Autodesk Inventor part; units mm, degrees
ref_plane "Piano di lavoro1" through (0, 13.85, 0) normal (0, 1, 0) x (1, 0, 0)
ref_plane "Piano di lavoro2" through (0, -10.75, 0) normal (0, -1, 0) x (1, 0, 0)
ref_plane "YZ Plane" through (0, 0, 0) normal (1, 0, 0) x (0, 1, 0)
sketch "Schizzo1" plane through (0, 0, 0) normal (0, 1, 0) x (-1, 0, 0)
  line L0 (-8.85, -43.18) -> (8.95, -43.18)
  line L1 (8.95, -43.18) -> (8.95, 17.78)
  line L2 (8.95, 17.78) -> (-8.85, 17.78)
  line L3 (-8.85, 17.78) -> (-8.85, -43.18)
  line L4 (-8.85, 17.78) -> (8.95, -43.18) construction
  line L5 (8.95, 17.78) -> (-8.85, -43.18) construction
  line L6 (8.95, 16.48) -> (-8.95, 16.48) construction
  line L7 (-7.6, 17.78) -> (-7.6, -43.18) construction
  circle A0 centre (-7.6, 16.48) radius 0.425
  circle A1 centre (-7.6, 13.94) radius 0.425
  circle A2 centre (-7.6, 11.4) radius 0.425
  circle A3 centre (-7.6, 8.86) radius 0.425
  circle A4 centre (-7.6, 6.32) radius 0.425
  circle A5 centre (-7.6, 3.78) radius 0.425
  circle A6 centre (-7.6, 1.24) radius 0.425
  circle A7 centre (-7.6, -1.3) radius 0.425
  circle A8 centre (-7.6, -3.84) radius 0.425
  circle A9 centre (-7.6, -6.38) radius 0.425
  circle A10 centre (-7.6, -8.92) radius 0.425
  circle A11 centre (-7.6, -11.46) radius 0.425
  circle A12 centre (-7.6, -14) radius 0.425
  circle A13 centre (-7.6, -16.54) radius 0.425
  circle A14 centre (-5.06, 16.48) radius 0.425
  circle A15 centre (-2.52, 16.48) radius 0.425
  circle A16 centre (0.02, 16.48) radius 0.425
  circle A17 centre (2.56, 16.48) radius 0.425
  circle A18 centre (5.1, 16.48) radius 0.425
  circle A19 centre (7.64, 16.48) radius 0.425
  circle A20 centre (7.64, 13.94) radius 0.425
  circle A21 centre (7.64, 11.4) radius 0.425
  circle A22 centre (7.64, 8.86) radius 0.425
  circle A23 centre (7.64, 6.32) radius 0.425
  circle A24 centre (7.64, 3.78) radius 0.425
  circle A25 centre (7.64, 1.24) radius 0.425
  circle A26 centre (7.64, -1.3) radius 0.425
  circle A27 centre (7.64, -3.84) radius 0.425
  circle A28 centre (7.64, -6.38) radius 0.425
  circle A29 centre (7.64, -8.92) radius 0.425
  circle A30 centre (7.64, -11.46) radius 0.425
  circle A31 centre (7.64, -14) radius 0.425
  circle A32 centre (7.64, -16.54) radius 0.425
  circle A33 centre (7.64, -19.08) radius 0.425
  circle A34 centre (7.64, -21.62) radius 0.425
  circle A35 centre (7.64, -24.16) radius 0.425
  circle A36 centre (7.64, -26.7) radius 0.425
  circle A37 centre (7.64, -29.24) radius 0.425
  circle A38 centre (7.64, -31.78) radius 0.425
  circle A39 centre (7.64, -34.32) radius 0.425
  circle A40 centre (7.64, -36.86) radius 0.425
  circle A41 centre (7.64, -39.4) radius 0.425
  circle A42 centre (7.64, -41.94) radius 0.425
  circle A43 centre (-7.6, -19.08) radius 0.425
  circle A44 centre (-7.6, -21.62) radius 0.425
  circle A45 centre (-7.6, -24.16) radius 0.425
  circle A46 centre (-7.6, -26.7) radius 0.425
  circle A47 centre (-7.6, -29.24) radius 0.425
  circle A48 centre (-7.6, -31.78) radius 0.425
  circle A49 centre (-7.6, -34.32) radius 0.425
  circle A50 centre (-7.6, -36.86) radius 0.425
  circle A51 centre (-7.6, -39.4) radius 0.425
  circle A52 centre (-7.6, -41.94) radius 0.425
  circle A53 centre (-5.06, -29.24) radius 0.425
  circle A54 centre (-2.52, -29.24) radius 0.425
  circle A55 centre (0.02, -29.24) radius 0.425
  circle A56 centre (2.56, -29.24) radius 0.425
  circle A57 centre (5.1, -29.24) radius 0.425
  point P0 (0, 0)
  point P1 (0.05, -12.7)
  dimension "d0" = 17.8
  dimension "d1" = 60.96
  dimension "d4" = 1.3
  dimension "d5" = 1.25
  dimension "d6" = 0.85
  dimension "d9" = 2.54
  dimension "d16" = 2.54
  dimension "d23" = 2.54
  dimension "d166" = 2.54
  dimension "d169" = 2.54
extrude "Estrusione2" add sketch "Schizzo1" along normal blind 1.6 contours L3 L2 L1 L0 | A14 | A15 | A16 | A17 | A18
fillet "Raccordo1" radius 0.2 12 edges at (-0.05, 0, 17.78) (-0.05, 1.6, 17.78) (8.85, 0.8, 17.78) (8.85, 0, -12.7) (8.85, 1.6, -12.7) (8.85, 0.8, -43.18) (-0.05, 0, -43.18) (-8.95, 0, -12.7) (-8.95, 0.8, -43.18) (-8.95, 0.8, 17.78) (-8.95, 1.6, -12.7) (-0.05, 1.6, -43.18)
ref_plane "Piano di lavoro1" through (0, 13.85, 0) normal (0, 1, 0) x (1, 0, 0)
sketch "Schizzo2" plane through (0, 13.85, 0) normal (0, 1, 0) x (1, 0, 0)
  line L0 (-8.9159, -19.3191) -> (-8.9159, 43.0633) construction
  line L1 (-8.9159, 43.0633) -> (8.8631, 43.0633) construction
  line L2 (8.8631, 43.0633) -> (8.8631, -19.3191) construction
  line L3 (8.8631, -19.3191) -> (-8.9159, -19.3191) construction
decal "Decalcomania1"
ref_plane "Piano di lavoro2" through (0, -10.75, 0) normal (0, -1, 0) x (1, 0, 0)
sketch "Schizzo3" plane through (0, -10.75, 0) normal (0, -1, 0) x (1, 0, 0)
  line L0 (9.0474, 17.6328) -> (9.0474, -44.6653) construction
  line L1 (9.0474, -44.6653) -> (-9.0191, -44.6653) construction
  line L2 (-9.0191, -44.6653) -> (-9.0191, 17.6328) construction
  line L3 (-9.0191, 17.6328) -> (9.0474, 17.6328) construction
  point P0 (0, 0)
decal "Decalcomania2"
sketch "Schizzo4" plane through (0, 1.6, 0) normal (0, 1, 0) x (1, 0, 0)
  circle A0 centre (7.6, 11.46) radius 0.425
sketch "Schizzo5" plane through (0, 1.6, 0) normal (0, 1, 0) x (1, 0, 0)
  circle A0 centre (7.6, -1.24) radius 0.425
sketch "Schizzo6" plane through (0, 1.6, 0) normal (0, 1, 0) x (1, 0, 0)
  circle A0 centre (7.6, -3.78) radius 0.425
sketch "Schizzo7" plane through (0, 1.6, 0) normal (0, 1, 0) x (1, 0, 0)
  circle A0 centre (-7.64, 16.54) radius 0.425
sketch "Schizzo8" plane through (0, 1.6, 0) normal (0, 1, 0) x (1, 0, 0)
  circle A0 centre (-7.64, 14) radius 0.425
sketch "Schizzo9" plane through (0, 1.6, 0) normal (0, 1, 0) x (1, 0, 0)
  circle A0 centre (-7.64, 11.46) radius 0.425
sketch "Sketch10" plane through (0, 0, 0) normal (0, -1, 0) x (1, 0, 0)
  circle A0 centre (7.6, -11.46) radius 0.425
sketch "Schizzo11" plane through (0, 0, 0) normal (0, -1, 0) x (1, 0, 0)
  circle A0 centre (-7.64, -16.54) radius 0.425
sketch "Schizzo12" plane through (0, 1.6, 0) normal (0, 1, 0) x (1, 0, 0)
  circle A0 centre (-7.64, -11.4) radius 0.425
sketch "Schizzo13" plane through (0, 1.6, 0) normal (0, 1, 0) x (1, 0, 0)
  circle A0 centre (-7.64, -8.86) radius 0.425
sketch "Schizzo14" plane through (0, 0, 0) normal (0, -1, 0) x (1, 0, 0)
  circle A0 centre (7.6, 1.24) radius 0.425
sketch "Schizzo15" plane through (0, 0, 0) normal (0, -1, 0) x (1, 0, 0)
  circle A0 centre (7.6, 3.78) radius 0.425
sketch "Sketch16" plane through (0, 0, 0) normal (0, -1, 0) x (1, 0, 0)
  point P0 (0, 0)
  point P1 (3.8313, 14.0194)
  point P2 (3.8313, 11.5063)
properties part number "101" material "Plastica ABS"
Source: CAD feature listing. Evaluate the final solid. Frame: model axes, mm. Coordinates: 2 decimals unless noted, no trailing zeros. Use a Markdown table: item, result. Add a question column.
Q1. Material intervals for L1, parallel to X at y = 1.1, z = -26.7 (3 decimals); L2, parallel to Z at x = -5, y = 1.2; L3, parallel to X at y = 0.9, z = 1, sorted ascending.
Q2. Section query A-A, the plane y = 0.5. State how many separate pieces and enclosed holes the cut face has, and give its area (3 significant figures).
Q3. Draft query along Y for faces 1 (the flat face through (0, 1.6, -12)), 2 (the flat face through (0, 0, -12)), 3 (the flat face through (0, 1, 17.78)). Return one class per face: pulls with the +Y half, pulls with the -Y half, needs draft (parallel to the pull), parting line crosses it, or undercut.
Result:
| question | item | result |
|---|---|---|
| 1 | L1 | x = -8.95 to -8.065, -7.215 to 7.175, 8.025 to 8.85 |
| 1 | L2 | z = -43.18 to -29.65, -28.83 to 17.78 |
| 1 | L3 | x = -8.95 to -7.99, -7.29 to 7.25, 7.95 to 8.85 |
| 2 | separate pieces | 1 |
| 2 | enclosed holes | 53 |
| 2 | area | 1,050 mm2 |
| 3 | face 1 | pulls with the +Y half |
| 3 | face 2 | pulls with the -Y half |
| 3 | face 3 | needs draft |
